from build123d import *

# Parameters (mm, degrees)
SKETCH1_W           = 40
SKETCH1_H           = 40
BOSS_EXTRUDE1_DEPTH = 40
SKETCH2_W           = 20
SKETCH2_H           = 10
CUT_EXTRUDE1_DEPTH  = 40
SKETCH3_W           = 20
SKETCH3_H           = 20
CUT_EXTRUDE2_DEPTH  = 40
SKETCH5_W           = 20
SKETCH5_H           = 20
CUT_EXTRUDE3_DEPTH  = 10
SKETCH7_W           = 20
SKETCH7_H           = 20
BOSS_EXTRUDE2_DEPTH = 10
SKETCH8_W           = 20
SKETCH8_H           = 20
BOSS_EXTRUDE3_DEPTH = 10
CUT_EXTRUDE10_DEPTH = 27
CUT_EXTRUDE12_DEPTH = 20
SKETCH12_W          = 20
SKETCH12_H          = 20
BOSS_EXTRUDE4_DEPTH = 0.0001
SKETCH14_W          = 9.999
SKETCH14_H          = 19.999
CUT_EXTRUDE19_DEPTH = 20.0001
CUT_EXTRUDE20_DEPTH = 20.0001
CUT_EXTRUDE21_DEPTH = 0.0001


with BuildPart() as part:
    # Sketch1 → Boss-Extrude1 (new body)
    with BuildSketch(Plane.XY):
        with Locations((20, 20)):
            Rectangle(SKETCH1_W, SKETCH1_H)
    extrude(amount=BOSS_EXTRUDE1_DEPTH)

    # Sketch2 → Cut-Extrude1 (cut)
    with BuildSketch(Plane(origin=(0, 40, 0), x_dir=(1, 0, 0), z_dir=(0, 1, 0))):
        with Locations((10, -35)):
            Rectangle(SKETCH2_W, SKETCH2_H)
    extrude(amount=-CUT_EXTRUDE1_DEPTH, mode=Mode.SUBTRACT)

    # Sketch3 → Cut-Extrude2 (cut)
    with BuildSketch(Plane.ZY):
        with Locations((30, 30)):
            Rectangle(SKETCH3_W, SKETCH3_H)
    extrude(amount=-CUT_EXTRUDE2_DEPTH, mode=Mode.SUBTRACT)

    # Sketch5 → Cut-Extrude3 (cut)
    with BuildSketch(Plane(origin=(40, 0, 0), x_dir=(0, 0, -1), z_dir=(1, 0, 0))):
        with Locations((-30, 10)):
            Rectangle(SKETCH5_W, SKETCH5_H)
    extrude(amount=-CUT_EXTRUDE3_DEPTH, mode=Mode.SUBTRACT)

    # Sketch7 → Boss-Extrude2 (add)
    with BuildSketch(Plane.XY.offset(20)):
        with Locations((10, 30)):
            Rectangle(SKETCH7_W, SKETCH7_H)
    extrude(amount=BOSS_EXTRUDE2_DEPTH)

    # Sketch8 → Boss-Extrude3 (add)
    with BuildSketch(Plane(origin=(30, 0, 0), x_dir=(0, 0, -1), z_dir=(1, 0, 0))):
        with Locations((-30, 10)):
            Rectangle(SKETCH8_W, SKETCH8_H)
    extrude(amount=BOSS_EXTRUDE3_DEPTH)

    # Sketch10 → Cut-Extrude10 (cut)
    with BuildSketch(Plane(origin=(0, 20, 0), x_dir=(1, 0, 0), z_dir=(0, 1, 0))):
        Polygon((20, -40), (40, -20), (40, -40), align=None)
    extrude(amount=-CUT_EXTRUDE10_DEPTH, mode=Mode.SUBTRACT)

    # Sketch11 → Cut-Extrude12 (cut)
    with BuildSketch(Plane.ZY):
        Polygon((10.0001, 39.9999), (0.0001, 0), (30.0001, 0), align=None)
    extrude(amount=-CUT_EXTRUDE12_DEPTH, mode=Mode.SUBTRACT)

    # Sketch12 → Boss-Extrude4 (add)
    with BuildSketch(Plane(origin=(0, 40, 0), x_dir=(1, 0, 0), z_dir=(0, 1, 0))):
        with Locations((30, -10)):
            Rectangle(SKETCH12_W, SKETCH12_H)
    extrude(amount=BOSS_EXTRUDE4_DEPTH)

    # Sketch14 → Cut-Extrude19 (cut)
    with BuildSketch(Plane.ZY):
        with Locations((25.0005, 30.0005)):
            Rectangle(SKETCH14_W, SKETCH14_H)
    extrude(amount=-CUT_EXTRUDE19_DEPTH, mode=Mode.SUBTRACT)

    # Sketch15 → Cut-Extrude20 (cut)
    with BuildSketch(Plane.ZY):
        Polygon((20.001, 20.001), (30, 20.001), (30, 0.0002), align=None)
    extrude(amount=-CUT_EXTRUDE20_DEPTH, mode=Mode.SUBTRACT)

    # Sketch16 → Cut-Extrude21 (cut)
    with BuildSketch(Plane.ZY.offset(-20)):
        Polygon((40, 20), (20.001, 20.001), (30, 0.0002), (40, 0), align=None)
    extrude(amount=-CUT_EXTRUDE21_DEPTH, mode=Mode.SUBTRACT)


solid = part.part
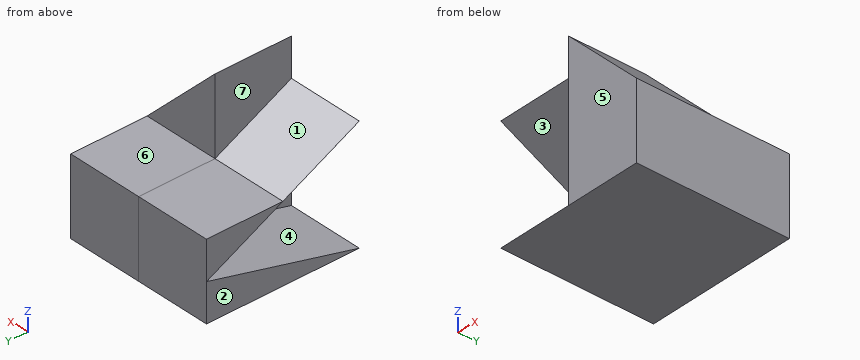
Geometry: final body of the model. Coordinates: model frame, mm. Face numbers are marked on the shaded views. A direction names the side the tool comes from. Coordinates: 2 decimals unless noted, no trailing zeros. Loops run counter-clockwise (first coordinate to the right, second up) from the corner with the lowest first, then second, coordinate; pieces in that order, holes last. Notation, with made-up numbers: (17.25, 33.25) - (24.25, 33.25) arc R28 cw to (24.25, 66.25) - close; hole circle Ø10 at (75, 80.5). An arc over 180 degrees is marked (long way). One line per question, with ' | ' between items. Start each with the question number.
(1) First-contact query: pin 1 (8 mm diameter, centred on x = 14.5, y = 8, fed in from +Z); pin 2 (1.5 mm diameter, centred on x = 14, y = 16.5, fed in from +Z); pin 3 (10 mm diameter, centred on x = 33, z = 33.5, fed in from +Y); pin 4 (2 mm diameter, centred on y = 31.5, z = 22, fed in from -X). Flat tips, straight axial feed; report the tip coordinate or a pass-through.
(2) Reachability of the marked faces 5, 6 and 7 from +Z, -Z, +X, -X, +Y, -Y: full face, straight path, thin tool, end or side. Return the list, or none.
(3) Ray query, L1, parallel to Z at x = 12.5, y = 26; L2, parallel to Z at x = 28, y = 21; L3, parallel to X at y = 7.5, z = 20. Return the intervals inside material, ascending. Write a range as from..to.
(4) Draft query along Z for the marked faces 1, 2, 3 and 4. Return one class per face: +Z half, -Z half, draft (parallel to the pull), parting line (faces both ways), or undercut.
(5) Cut plane D-D on x = 35. Output: boundary loops of the cut face in (y, z).
Here are the results:
1) pin 1: z = 28 | pin 2: z = 22.13 | pin 3: y = 20 | pin 4: through
2) face 5: +Z, -Z, +X, -X, -Y | face 6: +Z, +X, -X, +Y | face 7: +Z, -X, +Y
3) L1: 0..6.5, 17..20 | L2: 0..20 | L3: 20..40
4) face 1: +Z half | face 2: draft | face 3: undercut | face 4: undercut
5) outline: (0, 0) - (40, 0) - (40, 20) - (20, 20) - (20, 25) - (0, 25) - close
